Build history of the part. All positions in model axes, mm. Round coordinates to 2 decimals unless told otherwise and drop trailing zeros. Loops run counter-clockwise (first coordinate to the right, second up) from the corner with the lowest first, then second, coordinate; pieces in that order, holes last. Notation, with made-up numbers: M 82,21.25 L 136,21.25 A33 ccw 136,60.25 Z; hole C 62,41 d3. An arc over 180 degrees is marked long. One line per item, written item: value.
```python
from build123d import *

# Parameters (mm, degrees)
SKETCH1_W           = 58
SKETCH1_H           = 58
BOSS_EXTRUDE1_DEPTH = 10
SKETCH2_R           = 2.5
CUT_EXTRUDE1_DEPTH  = 10
SKETCH7_R           = 1.95
CUT_EXTRUDE4_DEPTH  = 43.213741838


with BuildPart() as part:
    # Sketch1 → Boss-Extrude1 (new body)
    with BuildSketch(Plane(origin=(0, 0, 0), x_dir=(1, 0, 0), z_dir=(0, 1, 0))):
        Rectangle(SKETCH1_W, SKETCH1_H)
    extrude(amount=BOSS_EXTRUDE1_DEPTH)

    # Sketch2 → Cut-Extrude1 (cut)
    with BuildSketch(Plane.ZY.offset(29)):
        with Locations((0, 5)):
            Circle(SKETCH2_R)
    extrude(amount=-CUT_EXTRUDE1_DEPTH, mode=Mode.SUBTRACT)

    # Sketch7 → Cut-Extrude4 (cut, through all)
    with BuildSketch(Plane(origin=(0, 10, 0), x_dir=(1, 0, 0), z_dir=(0, 1, 0))):
        with Locations(Location((-3.791486316, 8.606059277, 0), (0, 0, 270))):
            Circle(SKETCH7_R)
        with Locations(Location((6.955184511, 5.175961247, 0), (0, 0, 270))):
            Circle(SKETCH7_R)
        with Locations(Location((-7.044475248, -2.229902286, 0), (0, 0, 270))):
            Circle(SKETCH7_R)
        with Locations(Location((3.791486316, -5.482891218, 0), (0, 0, 270))):
            Circle(SKETCH7_R)
    extrude(amount=-CUT_EXTRUDE4_DEPTH, mode=Mode.SUBTRACT)


solid = part.part
```
Item 1: Slice it at B-B, the plane y = 5. Give the cut face in (x, z).
Check values:
outline: M -29,-29 L 29,-29 L 29,29 L -29,29 L -29,2.5 L -19,2.5 L -19,-2.5 L -29,-2.5 Z; hole C -7.04,2.23 d3.9; hole C -3.79,-8.61 d3.9; hole C 3.79,5.48 d3.9; hole C 6.96,-5.18 d3.9
Item 2: Wall check: line 1 along Z through (x, y) = (6.5, 9.75); line 2 along X through (y, z) = (5.75, -2); line 3 along Z through (x, y) = (-5, 4). Give the ranges that are in metal, low to high.
Check values:
line 1: z = -29 to -7.07, -3.28 to 29
line 2: x = -19 to 29
line 3: z = -29 to -10.14, -7.08 to 29
Item 3: Drop flat-ended pins along their axis: P1, Ø6, axis at x = -7.04, z = 2.23, coming from the +Y side; P2, Ø1.5, axis at y = 4.5, z = 1, coming from the -X side. Give the stop position or say it passes through.
Check values:
P1: stops at y = 10
P2: stops at x = -19
Item 4: Pull direction Y, two halves, no side cores. Call faces 1 (the face through (-19, 5, 0)), 2 (the face through (-24.07, 7.48, -0.33)), 3 (the face through (0, 10, 0)), 4 (the face through (-5.7, 5.1, -9)): pulls with the +Y half, pulls with the -Y half, needs draft (parallel to the pull), parting line crosses it, or undercut.
Check values:
face 1: undercut
face 2: undercut
face 3: pulls with the +Y half
face 4: needs draft
Item 5: Slice it at A-A, the plane z = 1. Give the cut face in (x, y).
Check values:
outline: M -29,0 L -8.56,0 L -8.56,10 L -29,10 L -29,7.29 L -19,7.29 L -19,2.71 L -29,2.71 Z; M -5.53,0 L 29,0 L 29,10 L -5.53,10 Z
